Input: dimensioned drawing with shaded views. Units: mm. Origin: part minimum x, y, z. A direction names the side the tool comes from. Coordinates: 2 decimals unless noted, no trailing zeros. Order: outer loops, then holes, each group sorted by start corner. A loop starts at its lowest first (then second) coordinate and runs counter-clockwise, first axis right, second up. Notation, with made-up numbers: M 56.25,31.5 L 81.25,31.5 A17 cw 81.25,54.5 Z; hole C 36,-25.75 d3. An arc over 180 degrees is marked long. Write item = value, one per line.
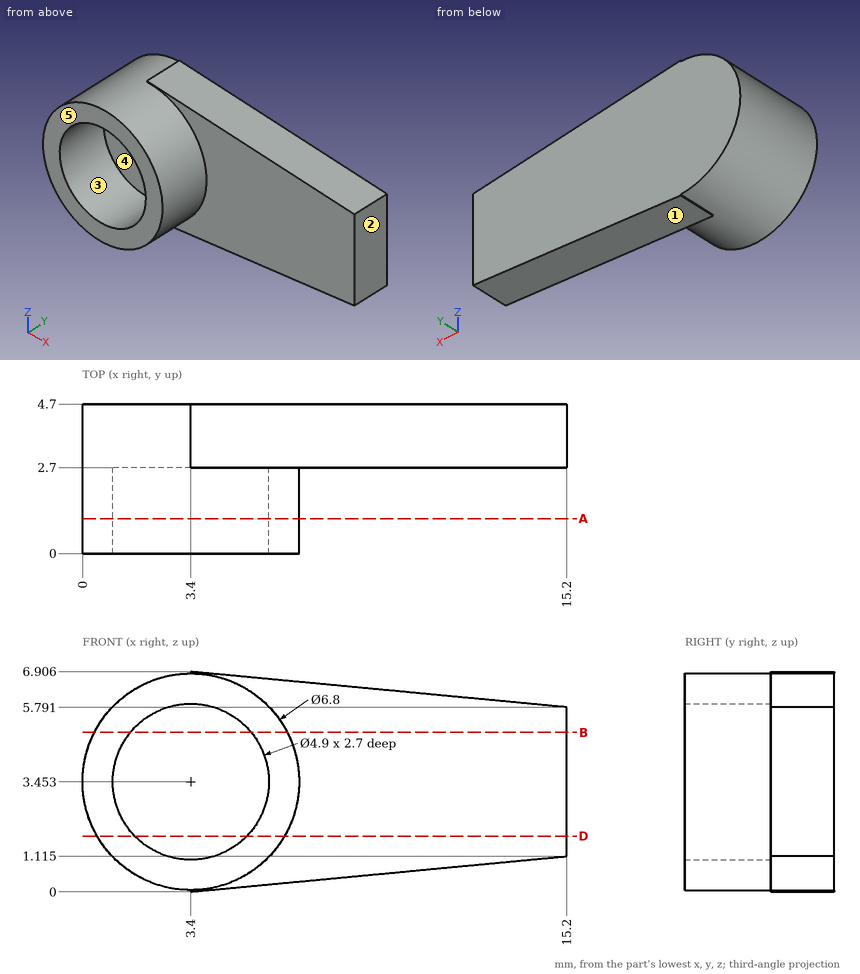
1) Mould query, pull axis Z, two halves, no side actions, for the marked faces 1, 2 and 3. Classes: pulls with the +Z half, pulls with the -Z half, needs draft (parallel to the pull), parting line crosses it, or undercut.
Numbers:
face_1 = pulls with the -Z half
face_2 = needs draft
face_3 = undercut
2) Section B-B, the plane z = 5. Return loops of the section in (x, y).
Numbers:
outline = M 0.37,0 L 1.5,0 L 1.5,2.7 L 5.3,2.7 L 5.3,0 L 6.43,0 L 6.43,2.7 L 15.2,2.7 L 15.2,4.7 L 0.37,4.7 Z
3) Line query: L1, parallel to X at y = 1, z = 3.5; L2, parallel to Y at x = 14, z = 1.75; L3, parallel to X at y = 1.3, z = 5.25 (1 decimal). Output: solid intervals per line, ascending.
Numbers:
L1 = 0 to 0.95, 5.85 to 6.8
L2 = 2.7 to 4.7
L3 = 0.5 to 1.7, 5.1 to 6.3
4) Section A-A, the plane y = 1.1. Return loops of the section in (x, z).
Numbers:
outline = C 3.4,3.45 d6.8; hole C 3.4,3.45 d4.9
5) Set-up query: the marked faces 4 and 5. Return all of +Z, -Z, +X, -X, +Y, -Y with unobstructed straight access to the full face (end or side cutting, diameter ignored); none if empty.
Numbers:
face_4 = -Y
face_5 = +Z, -Z, +X, -X, -Y
6) Section D-D, the plane z = 1.75. Return loops of the section in (x, y).
Numbers:
outline = M 0.46,0 L 1.64,0 L 1.64,2.7 L 5.16,2.7 L 5.16,0 L 6.34,0 L 6.34,2.7 L 15.2,2.7 L 15.2,4.7 L 0.46,4.7 Z
7) Pin query (flat end, axial travel): pin 1 (3.5 mm diameter, centred on x = 9.5, z = 5, fed in from -Y); pin 2 (1 mm diameter, centred on x = 8, y = 3.5, fed in from -Z); pin 3 (1.5 mm diameter, centred on y = 1.5, z = 2, fed in from +X). Return the tip coordinate at first contact, or that it passes through.
Numbers:
pin_1 = 2.7
pin_2 = 0.39
pin_3 = 6.73
